Drawing for the job (mm, zero at the part's lowest x, y, z). Round coordinates to 2 decimals unless told otherwise and drop trailing zeros. Loops run counter-clockwise (first coordinate to the right, second up) from the corner with the lowest first, then second, coordinate; pieces in that order, holes last. Notation, with made-up numbers: (76.25, -31.5) - (131.25, -31.5) arc R21 ccw to (131.25, 3.5) - close; hole circle Ø11 at (-31.5, 33). An arc over 180 degrees is marked (long way). Put each result on its own line as item: value.
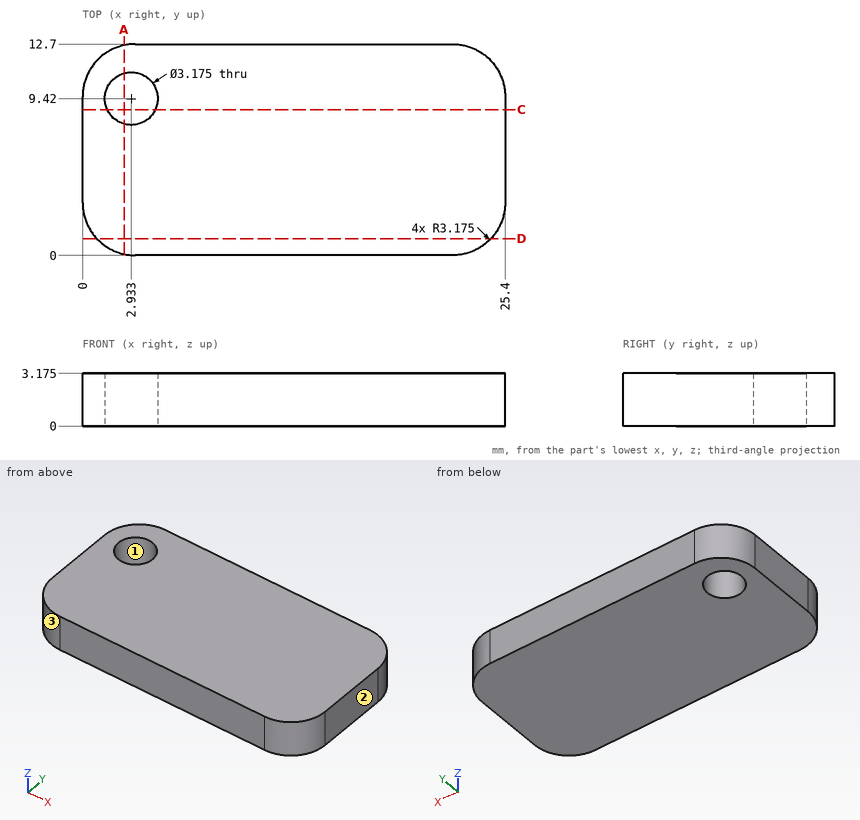
1. Probe line 1 along Y through (x, z) = (1.75, 0.45); line 2 along Y through (x, z) = (2.25, 1.45) (1 decimal); line 3 along Y through (x, z) = (24.25, 0.7). List the from-to ranges inside material, lowest first. Write a range as [from, to].
A:
line 1: y = [0.34, 8.36], [10.48, 12.36]
line 2: y = [0.1, 8], [10.9, 12.6]
line 3: y = [0.73, 11.97]
2. Band-saw the part on D-D (y = 1). List the corners of the cut face in (x, z) (1 decimal).
A:
outline: (0.9, 0) - (24.5, 0) - (24.5, 3.2) - (0.9, 3.2) - close
3. Band-saw the part on C-C (y = 8.75). List the corners of the cut face in (x, z) (1 decimal).
A:
outline: (0, 0) - (1.5, 0) - (1.5, 3.2) - (0, 3.2) - close; (4.4, 0) - (25.4, 0) - (25.4, 3.2) - (4.4, 3.2) - close
4. Band-saw the part on A-A (x = 2.5). List the corners of the cut face in (y, z) (1 decimal).
A:
outline: (0.1, 0) - (7.9, 0) - (7.9, 3.2) - (0.1, 3.2) - close; (10.9, 0) - (12.6, 0) - (12.6, 3.2) - (10.9, 3.2) - close
5. Two-plate mould, pull along Y, no slides. Class the marked faces 1, 2 and 3: pulls with the +Y half, pulls with the -Y half, needs draft (parallel to the pull), parting line crosses it, or undercut.
A:
face 1: undercut
face 2: needs draft
face 3: pulls with the -Y half
